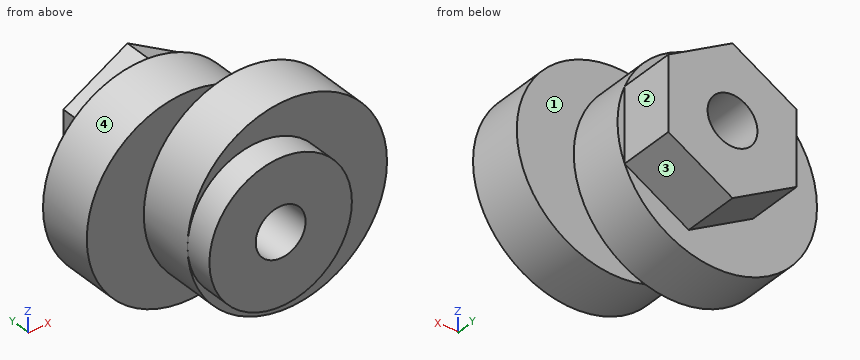
```python
from build123d import *

# Parameters (mm, degrees)
SKETCH1_R           = 5
BOSS_EXTRUDE1_DEPTH = 2
SKETCH2_R           = 7
BOSS_EXTRUDE2_DEPTH = 4
SKETCH4_R           = 7
BOSS_EXTRUDE4_DEPTH = 4
SKETCH5_R           = 1.75
CUT_EXTRUDE1_DEPTH  = 11
SKETCH6_R           = 1.75
BOSS_EXTRUDE5_DEPTH = 4


with BuildPart() as part:
    # Sketch1 → Boss-Extrude1 (new body)
    with BuildSketch(Plane(origin=(0, 0, 0), x_dir=(1, 0, 0), z_dir=(0, 1, 0))):
        Circle(SKETCH1_R)
    extrude(amount=BOSS_EXTRUDE1_DEPTH)

    # Sketch2 → Boss-Extrude2 (add)
    with BuildSketch(Plane(origin=(0, 2, 0), x_dir=(1, 0, 0), z_dir=(0, 1, 0))):
        with Locations((2, 0)):
            Circle(SKETCH2_R)
    extrude(amount=BOSS_EXTRUDE2_DEPTH)

    # Sketch4 → Boss-Extrude4 (add)
    with BuildSketch(Plane(origin=(0, 6, 0), x_dir=(1, 0, 0), z_dir=(0, 1, 0))):
        with Locations((-2, 0)):
            Circle(SKETCH4_R)
    extrude(amount=BOSS_EXTRUDE4_DEPTH)

    # Sketch5 → Cut-Extrude1 (cut, through all)
    with BuildSketch(Plane.XZ):
        Circle(SKETCH5_R)
    extrude(amount=-CUT_EXTRUDE1_DEPTH, mode=Mode.SUBTRACT)

    # Sketch6 → Boss-Extrude5 (add)
    with BuildSketch(Plane(origin=(0, 10, 0), x_dir=(1, 0, 0), z_dir=(0, 1, 0))):
        Polygon((-4.5, 2.598076211), (-4.5, -2.598076211), (0, -5.196152423), (4.5, -2.598076211), (4.5, 2.598076211), (0, 5.196152423), align=None)
        Circle(SKETCH6_R, mode=Mode.SUBTRACT)
    extrude(amount=BOSS_EXTRUDE5_DEPTH)


solid = part.part
```
Could you check a few things on this model? Use its own coordinates, in mm. Face numbers are marked on the shaded views. A direction names the side the tool comes from. Give positions to 0.01 mm unless a question says otherwise; leave off trailing zeros. Loops run counter-clockwise (first coordinate to the right, second up) from the corner with the lowest first, then second, coordinate; pieces in that order, holes last. Notation, with made-up numbers: (35.25, 75) - (62.25, 75) arc R33 cw to (62.25, 110) - close; hole circle Ø11 at (-7.75, 35). An arc over 180 degrees is marked (long way). Answer in a Markdown table with one row per item. Add a question column.
Q1. If we section it at C-C (z = 6): List the corners of the cut face in (x, y) for me.
Q2. For pin 1 (5 mm diameter, centred on y = 1.5, z = 5, fed in from -X); pin 2 (2 mm diameter, centred on y = 7, z = -4, fed in from -X); pin 3 (3 mm diameter, centred on y = 12, z = 0, fed in from +X); pin 4 (4 mm diameter, centred on x = 2, z = -0.5, fed in from -Y), each with a flat end and sliding along its axis, tell me the tip position at first contact or that it passes through.
Q3. Please list where these lines run through material, in increasing order: L1, parallel to X at y = 4, z = 0; L2, parallel to Y at x = -7.5, z = 2.25; L3, parallel to Y at x = 5.25, z = -2.5. Write a range as from..to.
Q4. If we section it at B-B (y = 8): List the corners of the cut face in (x, z) for me, plus the area to 3 significant figures.
Q5. If we section it at D-D (x = 5.75): List the corners of the cut face in (y, z) for me.
Q6. Which directions (+Z, -Z, +X, -X, +Y, -Y) give clear straight access to the entire face, cutting with the end or side of a thin tool? Please do the marked faces 1, 2, 3 and 4.
Q7. If we section it at A-A (x = -0.5): List the corners of the cut face in (y, z) for me.
The answers:
| question | item | result |
|---|---|---|
| 1 | outline | (-5.61, 6) - (-1.61, 6) - (-1.61, 2) - (5.61, 2) - (5.61, 6) - (1.61, 6) - (1.61, 10) - (-5.61, 10) - close |
| 2 | pin 1 | stops at x = -4.52 |
| 2 | pin 2 | stops at x = -8.32 |
| 2 | pin 3 | stops at x = 4.5 |
| 2 | pin 4 | stops at y = 0 |
| 3 | L1 | x = -5..-1.75, 1.75..9 |
| 3 | L2 | y = 6..10 |
| 3 | L3 | y = 2..6 |
| 4 | outline | circle Ø14 at (-2, 0); hole circle Ø3.5 at (0, 0) |
| 4 | area | 144 mm^2 |
| 5 | outline | (2, -5.91) - (6, -5.91) - (6, 5.91) - (2, 5.91) - close |
| 6 | face 1 | +X, +Y |
| 6 | face 2 | +Z, -Z, +X, +Y |
| 6 | face 3 | -Z, +X, +Y |
| 6 | face 4 | +Y |
| 7 | outline | (0, -4.97) - (2, -4.97) - (2, -6.54) - (6, -6.54) - (6, -6.84) - (10, -6.84) - (10, -4.91) - (14, -4.91) - (14, -1.68) - (0, -1.68) - close; (0, 1.68) - (14, 1.68) - (14, 4.91) - (10, 4.91) - (10, 6.84) - (6, 6.84) - (6, 6.54) - (2, 6.54) - (2, 4.97) - (0, 4.97) - close |
